```python
from build123d import *

# Parameters (mm, degrees)
SM_BASE_FLANGE_1_DEPTH   = 4
OTHER_START              = -11.5
OTHER_2_DEPTH            = 4
CUT_EXTRUDE_1_DEPTH      = 126.982552614
CUT_EXTRUDE_1_DEPTH_BACK = 126.982552614
SKETCH_7_W               = 3.023259835
SKETCH_7_H               = 4


# Read off the part's stored shape, not the designer's step: Полость2
# Sheet-metal steps are written as plain solids
with BuildPart() as part:
    # Sketch 2 → Базовая кромка1 (new body)
    with BuildSketch(Plane(origin=(0, 0, 0), x_dir=(1, 0, 0), z_dir=(0, 1, 0))):
        Polygon((41, 0), (-70.990165257, 0), (-30, 104), (0, 104), align=None)
    extrude(amount=SM_BASE_FLANGE_1_DEPTH)

    # Полость2 outline → Полость2 (cut)
    with BuildSketch(Plane.XY.offset(OTHER_START)):
        Polygon((-70, 0), (-3, 0), (-6.023259835, 4), (-70, 4), align=None)
    extrude(amount=OTHER_2_DEPTH, mode=Mode.SUBTRACT)

    # Эскиз7 → Вырез-Вытянуть1 (cut, two sides: drawn at the far end of the back side and taken through both)
    with BuildSketch(Plane(origin=(0, 4, 0), x_dir=(1, 0, 0), z_dir=(0, 1, 0)).offset(-CUT_EXTRUDE_1_DEPTH_BACK)):
        with Locations((-4.511629918, 9.5)):
            Rectangle(SKETCH_7_W, SKETCH_7_H)
    extrude(amount=CUT_EXTRUDE_1_DEPTH + CUT_EXTRUDE_1_DEPTH_BACK, mode=Mode.SUBTRACT)


solid = part.part
```
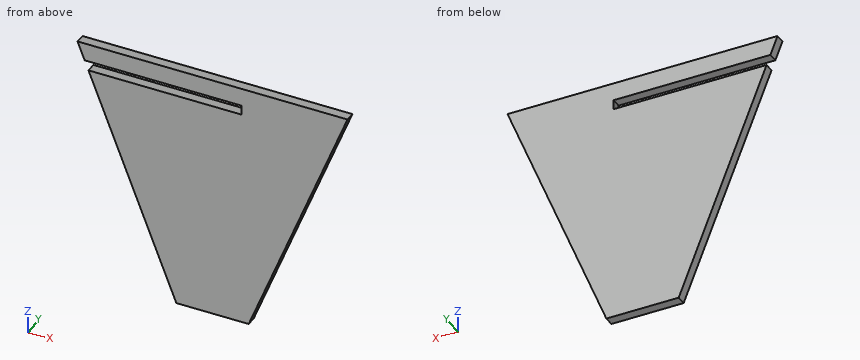
Geometry check sheet. Reference: the model listing, model coordinates, mm. Give positions to 0.01 mm unless a question says otherwise; leave off trailing zeros. Order: outer loops, then holes, each group sorted by start corner. A loop starts at its lowest first (then second) coordinate and runs counter-clockwise, first axis right, second up.
1. Gauge pin test, flat ends, axial feed: pin 1 Ø2 at (y, z) = (1.5, -32.5) entering from +X; pin 2 Ø2 at (y, z) = (0.5, -85.5) entering from +X; pin 3 Ø1 at (y, z) = (3, -58.5) entering from -X. Record the tip position at first contact, or that the pin passes through.
2. Section check C-C, the plane x = -42. Enter the section's corners in (y, z), and give its area (3 significant figures).
3. Section check A-A, the plane x = -21. Enter the section's corners in (y, z).
4. Section check D-D, the plane z = -24. Enter the section's corners in (x, y), and give its area (3 significant figures).
5. Thickness scan on L1, parallel to Z at x = -22, y = 3.7; L2, parallel to X at y = 3.85, z = -60; L3, parallel to X at y = 0.35, z = -4. Record the ranges inside material, lowest first.
6. Section check B-B, the plane y = 1.75. Enter the section's corners in (x, z).
Values follow:
1. pin 1: stops at x = 28.58
1. pin 2: stops at x = 7.69
1. pin 3: stops at x = -48.13
2. outline: (0, -73.55) - (4, -73.55) - (4, -11.5) - (0, -11.5) - close; (0, -7.5) - (4, -7.5) - (4, 0) - (0, 0) - close
2. area: 278 mm2
3. outline: (0, -104) - (4, -104) - (4, -11.5) - (0, -11.5) - close; (0, -7.5) - (4, -7.5) - (4, 0) - (0, 0) - close
4. outline: (-61.53, 0) - (31.54, 0) - (31.54, 4) - (-61.53, 4) - close
4. area: 372 mm2
5. L1: z = -104 to -11.5, -7.5 to 0
5. L2: x = -47.34 to 17.35
5. L3: x = -69.41 to 39.42
6. outline: (-70.99, 0) - (-68.03, -7.5) - (-3, -7.5) - (-3, -11.5) - (-66.46, -11.5) - (-30, -104) - (0, -104) - (41, 0) - close
